Input: part model. Units: mm. Frame: model coordinates. A direction names the side the tool comes from. Round coordinates to 2 decimals unless told otherwise and drop trailing zeros. Order: outer loops, then holes, each group sorted by start corner. A loop starts at its lowest first (then second) coordinate and runs counter-clockwise, first axis right, second up. Notation, with made-up numbers: M 33,15.5 L 55,15.5 A25 ccw 55,39.5 Z; hole C 6.5,27.25 d8. An arc over 180 degrees is marked long. One line per question, with ' | ' between items.
```python
from build123d import *

# Parameters (mm, degrees)
PAD_DEPTH    = 3.7
SKETCH001_W  = 0.5
SKETCH001_H  = 5.5
PAD001_DEPTH = 0.19


with BuildPart() as pad:
    # Sketch002 → Pad (new body)
    with BuildSketch(Plane.XY.offset(2.5)):
        Polygon((1.11, 1.54), (3.97, 1.54), (4.54, 0), (4.4, -0.77), (0.68, -0.77), (0.54, 0), align=None)
    extrude(amount=PAD_DEPTH)


with BuildPart() as to_92s_wide:
    # Sketch001 → Pad001 (new body, symmetric)
    with BuildSketch(Plane.XZ):
        with Locations((2.54, 0.05)):
            Rectangle(SKETCH001_W, SKETCH001_H)
        Polygon((0.25, -2.7), (-0.25, -2.7), (-0.25, 0.26), (1.02, 2.16), (1.02, 2.8), (1.52, 2.8), (1.52, 2.16), (0.25, 0.26), align=None)
        Polygon((3.56, 2.8), (4.06, 2.8), (4.06, 2.16), (5.33, 0.26), (5.33, -2.7), (4.83, -2.7), (4.83, 0.26), (3.56, 2.16), align=None)
    extrude(amount=PAD001_DEPTH, both=True)

    add(pad.part)


solid = to_92s_wide.part
```
Item 1: First-contact query: pin 1 (1.9 mm diameter, centred on x = 1, z = 0, fed in from -Y); pin 2 (1.2 mm diameter, centred on x = 2, y = 1, fed in from -Z); pin 3 (1.4 mm diameter, centred on x = 0.5, z = -0.5, fed in from +Y). Flat tips, straight axial feed; report the tip coordinate or a pass-through.
Report:
pin 1: y = -0.19 | pin 2: z = 2.5 | pin 3: y = 0.19
Item 2: Section query A-A, the plane z = 1.25. Return loops of the section in (x, y), plus the area to 3 significant figures.
Report:
outline: M 0.41,-0.19 L 0.91,-0.19 L 0.91,0.19 L 0.41,0.19 Z; M 2.29,-0.19 L 2.79,-0.19 L 2.79,0.19 L 2.29,0.19 Z; M 4.17,-0.19 L 4.67,-0.19 L 4.67,0.19 L 4.17,0.19 Z | area: 0.570 mm²
Item 3: Mould query, pull axis X, two halves, no side actions, for faces 4 (the flat face through (4.25, 0.78, 4.32)), 5 (the flat face through (5, 0.19, 0)), 6 (the flat face through (4.2, 0, 1.2)). Classes: +X half, -X half, draft (parallel to the pull), parting line (faces both ways), or undercut.
Report:
face 4: +X half | face 5: draft | face 6: undercut
Item 4: Line query: line 1 along X through (y, z) = (-0.15, -1.25); line 2 along Z through (x, y) = (2.55, 0.25); line 3 along Y through (x, z) = (4.5, 1.25). Output: solid intervals per line, ascending. Write a range as from..to.
Report:
line 1: -0.25..0.25, 2.29..2.79, 4.83..5.33 | line 2: 2.5..6.2 | line 3: -0.19..0.19
Item 5: Section query C-C, the plane y = 0.1. Return loops of the section in (x, z), plus the area to 3 significant figures.
Report:
outline: M -0.25,-2.7 L 0.25,-2.7 L 0.25,0.26 L 1.52,2.16 L 1.52,2.5 L 2.29,2.5 L 2.29,-2.7 L 2.79,-2.7 L 2.79,2.5 L 3.56,2.5 L 3.56,2.16 L 4.83,0.26 L 4.83,-2.7 L 5.33,-2.7 L 5.33,0.26 L 4.06,2.16 L 4.06,2.5 L 4.5,2.5 L 4.5,6.2 L 0.58,6.2 L 0.58,2.5 L 1.02,2.5 L 1.02,2.16 L -0.25,0.26 Z | area: 22.3 mm²
Item 6: Access query for faces 1 (the flat face through (0, 0.19, 0)), 2 (the flat face through (5, -0.19, 0)), 3 (the flat face through (4.7, 0, 1.2)). Directions: +Z, -Z, +X, -X, +Y, -Y. A direction counts if a zero-diameter tool reaches every point of the face in a straight line with its end or side. Return the directions, or none.
Report:
face 1: -Z, +X, -X, +Y | face 2: -Z, +X, -X, -Y | face 3: +X, +Y, -Y
Item 7: Section query D-D, the plane x = 2.1. Return loops of the section in (y, z), plus the area to 3 significant figures.
Report:
outline: M -0.77,2.5 L 1.54,2.5 L 1.54,6.2 L -0.77,6.2 Z | area: 8.55 mm²
Item 8: Section query B-B, the plane z = 4.5. Return loops of the section in (x, y), plus the area to 3 significant figures.
Report:
outline: M 0.54,0 L 0.68,-0.77 L 4.4,-0.77 L 4.54,0 L 3.97,1.54 L 1.11,1.54 Z | area: 8.25 mm²
